```python
from build123d import *

# Parameters (mm, degrees)
F0_R      = 10
F1_DEPTH  = 10
F3_DEPTH  = 10
F4_R      = 9
F5_DEPTH  = 5
F7_DEPTH  = 5
F8_R      = 9
F9_DEPTH  = 5
F11_DEPTH = 10
F12_R     = 10
F13_DEPTH = 5
F14_R     = 7.5
F14_R_2   = 6
F16_DEPTH = 26


with BuildPart() as f1:
    # F0 (on Front) → F1 (new body, symmetric)
    with BuildSketch(Plane.XZ):
        Circle(F0_R)
    extrude(amount=F1_DEPTH, both=True)

    # F2 (on face) → F3 (join)
    with BuildSketch(Plane.XZ.offset(10)):
        Polygon((4.264543, -11.964406), (12.493751, -2.289001), (8.229208, 9.675405), (-4.264543, 11.964406), (-12.493751, 2.289001), (-8.229208, -9.675405), align=None)
    extrude(amount=F3_DEPTH)

    # F4 (on face) → F5 (join)
    with BuildSketch(Plane.XZ.offset(20)):
        Circle(F4_R)
    extrude(amount=F5_DEPTH)

    # F6 (on face) → F7 (join)
    with BuildSketch(Plane.XZ.offset(25)):
        Polygon((5.858879, -9.95022), (11.546582, 0.098828), (5.687704, 10.049048), (-5.858879, 9.95022), (-11.546582, -0.098828), (-5.687704, -10.049048), align=None)
    extrude(amount=F7_DEPTH)

    # F8 (on face) → F9 (join)
    with BuildSketch(Plane.XZ.offset(30)):
        Circle(F8_R)
    extrude(amount=F9_DEPTH)

    # F10 (on face) → F11 (join)
    with BuildSketch(Plane.XZ.offset(35)):
        Polygon((8.229208, 9.675405), (-4.264543, 11.964406), (-12.493751, 2.289001), (-8.229208, -9.675405), (4.264543, -11.964406), (12.493751, -2.289001), align=None)
    extrude(amount=F11_DEPTH)

    # F12 (on face) → F13 (join)
    with BuildSketch(Plane.XZ.offset(45)):
        Circle(F12_R)
    extrude(amount=F13_DEPTH)

    # F14 (on face) → F16 (join, through all)
    with BuildSketch(Plane.XZ.offset(50)):
        Circle(F14_R)
        Circle(F14_R_2, mode=Mode.SUBTRACT)
    extrude(amount=F16_DEPTH)


solid = f1.part
```
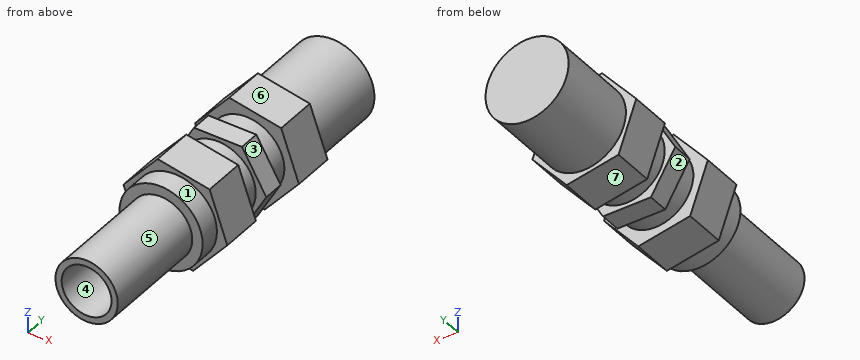
Check sheet for the modelled part. Datum: model origin and axes. Units: mm. Face numbers are marked on the shaded views. A direction names the side the tool comes from. Coordinates: 2 decimals unless noted, no trailing zeros. Order: outer loops, then holes, each group sorted by start corner. A loop starts at its lowest first (then second) coordinate and runs counter-clockwise, first axis right, second up. Notation, with made-up numbers: (59.5, 18.25) -> (97.5, 18.25) arc R21 ccw to (97.5, 28.25) -> close; hole circle Ø11 at (-28.75, -11.75). An arc over 180 degrees is marked (long way). Write item = value, one per line. Start each with the question number.
1) Cross-section at A-A (y = -26.5). Enter the section's corners in (x, z).
2) Material ranges on L1, parallel to Y at x = 1.25, z = 9.5; L2, parallel to Z at x = 0, y = -63; L3, parallel to Y at x = -3, z = -0.5, recorded low to high.
3) Mould release check, pull along Z, two halves, no side actions. Record for the marked faces 4, 5, 6 and 7: +Z half, -Z half, draft (parallel to the pull), parting line (faces both ways), or undercut.
4) Go/stop test with flat-tipped pins: P1, Ø8, axis at y = -16, z = -8.5, coming from the -X side; P2, Ø8, axis at y = -51, z = 7.5, coming from the +X side; P3, Ø5, axis at y = -40.5, z = 2.5, coming from the +X side. Record where each tip stops, or that it passes through.
5) Cross-section at B-B (y = -63.5). Enter the section's corners in (x, z).
6) Cross-section at C-C (y = 1). Enter the section's corners in (x, z), then the cut area to 3 significant figures.
7) Access from +Z, -Z, +X, -X, +Y, -Y to the whole of each face (thin tool, end or side, straight path). Record for the marked faces 1, 2 and 3.
Ans:
q1.outline = (-11.55, -0.1) -> (-5.69, -10.05) -> (5.86, -9.95) -> (11.55, 0.1) -> (5.69, 10.05) -> (-5.86, 9.95) -> close
q2.L1 = -50 to -35, -30 to -25, -20 to 10
q2.L2 = -7.5 to -6, 6 to 7.5
q2.L3 = -50 to 10
q3.face_4 = undercut
q3.face_5 = parting line
q3.face_6 = +Z half
q3.face_7 = -Z half
q4.P1 = -10.07
q4.P2 = 9.32
q4.P3 = 11.68
q5.outline = circle Ø15 at (0, 0); hole circle Ø12 at (0, 0)
q6.outline = circle Ø20 at (0, 0)
q6.area = 314 mm²
q7.face_1 = -Y
q7.face_2 = -Z, -X
q7.face_3 = +Z, +X
